Here's how the part is built. I have some questions about the finished solid (model axes, mm). Face numbers are marked on the shaded views. A direction names the side the tool comes from. Coordinates: 2 decimals unless noted, no trailing zeros. Order: outer loops, then holes, each group sorted by start corner. A loop starts at its lowest first (then second) coordinate and runs counter-clockwise, first axis right, second up. Notation, with made-up numbers: (45, 14) -> (80, 14) arc R27 ccw to (80, 49) -> close; hole circle Ø5 at (2, 20). An arc over 180 degrees is marked (long way). One line per item, written item: value. Start each with the question number.
```python
from build123d import *

# Parameters (mm, degrees)
ESQUISSE2_R      = 2.6
EXTRUSION1_DEPTH = 3.12
EXTRUSION2_START = -10
ESQUISSE4_R      = 2.6
EXTRUSION2_DEPTH = 10
CONG_1_R         = 0.2
CHANFREIN1_SIZE  = 0.4


with BuildPart() as part:
    # Esquisse2 → Extrusion1 (new body)
    with BuildSketch(Plane.XY):
        Polygon((6.92820323, 0), (3.464101615, 6), (-3.464101615, 6), (-6.92820323, 0), (-3.464101615, -6), (3.464101615, -6), align=None)
        with Locations(Location((0, 0, 0), (0, 0, 180))):
            Circle(ESQUISSE2_R, mode=Mode.SUBTRACT)
    extrude(amount=EXTRUSION1_DEPTH)

    # Esquisse3 → Révolution1 (revolve)
    with BuildSketch(Plane(origin=(0, 0, 0), x_dir=(1, 0, 0), z_dir=(0, 1, 0))):
        with BuildLine():
            Line((5.5, 0), (0, 0))
            Line((0, 0), (0, 10.78))
            ThreePointArc((0, 10.78), (1.326705119, 10.462857182), (2.366555702, 9.58))
            ThreePointArc((2.366555702, 9.58), (4.696738417, 5.039714108), (5.5, 0))
        make_face()
    revolve(axis=Axis((0, 0, 0), (0, 0, -1)))

    # Esquisse4 → Extrusion2 (cut)
    with BuildSketch(Plane.XY.offset(3.12).offset(EXTRUSION2_START)):
        with Locations(Location((0, 0, 0), (0, 0, 180))):
            Circle(ESQUISSE4_R)
    extrude(amount=EXTRUSION2_DEPTH, mode=Mode.SUBTRACT)

    # Congé1
    cong_1_edges = [part.edges().sort_by_distance(p)[0] for p in [
        (-3.464101615, -6, 1.56),
        (-6.92820323, 0, 1.56),
        (-3.464101615, 6, 1.56),
        (3.464101615, 6, 1.56),
        (6.92820323, 0, 1.56),
        (3.464101615, -6, 1.56),
    ]]
    fillet(cong_1_edges, radius=CONG_1_R)

    # Chanfrein1
    chanfrein1_edges = [part.edges().sort_by_distance(p)[0] for p in [
        (2.6, 0, 3.12),
    ]]
    chamfer(chanfrein1_edges, length=CHANFREIN1_SIZE)


solid = part.part
```
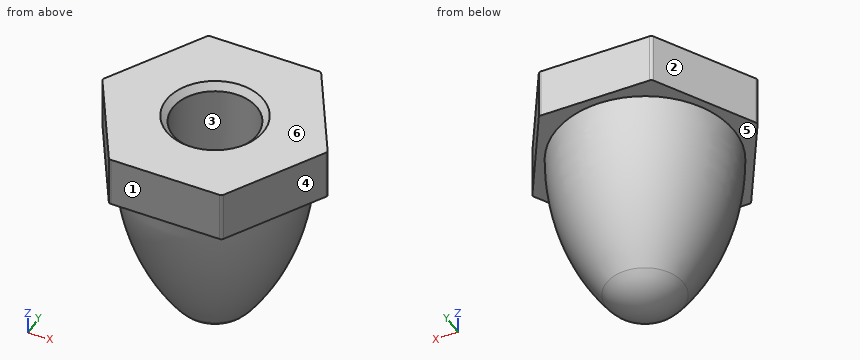
Q1. I need wall thicknesses on line 1 (Y direction, x = 0, z = -1.25); line 2 (Y direction, x = 0, z = -3); line 3 (Y direction, x = 3.75, z = 2). Which ranges of each line are inside material? Lowest first, please.
Q2. If we mould it in two halves opening along X, with no side actions, what happens to the marked faces 1, 2, 3 and 4? For each: +X half, -X half, draft (parallel to the pull), parting line (faces both ways), or undercut.
Q3. Imagine slicing it at A-A (z = 2.25). Write out the boundary of the cut face in (x, y), plus the area to 3 significant figures.
Q4. For P1, Ø1.6, axis at x = 0, y = 1.5, coming from the +Z side; P2, Ø4, axis at y = 1.5, z = -4, coming from the +X side; P3, Ø1, axis at x = 3.5, z = -6, coming from the +Y side, each with a flat end and sliding along its axis, tell me the tip position at first contact or that it passes through.
Q5. For the marked faces 5 and 6, which set-ups out of +Z, -Z, +X, -X, +Y, -Y let a thin tool reach every point of the face, with its end or its side?
Completed:
1. line 1: y = -5.45 to -2.6, 2.6 to 5.45
1. line 2: y = -5.22 to -2.6, 2.6 to 5.22
1. line 3: y = -5.5 to 5.5
2. face 1: draft
2. face 2: -X half
2. face 3: undercut
2. face 4: +X half
3. outline: (-6.87, -0.1) -> (-3.52, -5.9) arc R0.2 ccw to (-3.35, -6) -> (3.35, -6) arc R0.2 ccw to (3.52, -5.9) -> (6.87, -0.1) arc R0.2 ccw to (6.87, 0.1) -> (3.52, 5.9) arc R0.2 ccw to (3.35, 6) -> (-3.35, 6) arc R0.2 ccw to (-3.52, 5.9) -> (-6.87, 0.1) arc R0.2 ccw to start; hole circle Ø5.2 at (0, 0)
3. area: 103 mm2
4. P1: stops at z = -6.88
4. P2: stops at x = 5.32
4. P3: stops at y = 3.22
5. face 5: -Z
5. face 6: +Z, +X, -X, +Y, -Y
